from build123d import *

# Parameters (mm, degrees)
BOSS_EXTRUDE1_DEPTH   = 25.4
SKETCH2_R             = 3.5
CUT_EXTRUDE1_DEPTH    = 84.762252835
SKETCH3_R             = 13.335
CUT_EXTRUDE2_DEPTH    = 5.08
SKETCH4_R             = 22.86
CUT_EXTRUDE3_DEPTH    = 5.08
F_4_CLEARANCE_HOLE1_D = 3.2639


with BuildPart() as part:
    # Sketch1 → Boss-Extrude1 (new body)
    with BuildSketch(Plane.XY):
        with BuildLine():
            Line((-8.980256121, 56.44003455), (0, 47.459778429))
            Line((0, 47.459778429), (8.980256121, 56.44003455))
            ThreePointArc((8.980256121, 56.44003455), (21.87035816, 52.799715283), (33.559131161, 46.259131161))
            Line((33.559131161, 46.259131161), (33.559131161, 33.559131161))
            Line((33.559131161, 33.559131161), (46.259131161, 33.559131161))
            ThreePointArc((46.259131161, 33.559131161), (52.799715283, 21.87035816), (56.44003455, 8.980256121))
            Line((56.44003455, 8.980256121), (47.459778429, 0))
            Line((47.459778429, 0), (56.44003455, -8.980256121))
            ThreePointArc((56.44003455, -8.980256121), (52.799715283, -21.87035816), (46.259131161, -33.559131161))
            Line((46.259131161, -33.559131161), (33.559131161, -33.559131161))
            Line((33.559131161, -33.559131161), (33.559131161, -46.259131161))
            ThreePointArc((33.559131161, -46.259131161), (21.87035816, -52.799715283), (8.980256121, -56.44003455))
            Line((8.980256121, -56.44003455), (0, -47.459778429))
            Line((0, -47.459778429), (-8.980256121, -56.44003455))
            ThreePointArc((-8.980256121, -56.44003455), (-21.87035816, -52.799715283), (-33.559131161, -46.259131161))
            Line((-33.559131161, -46.259131161), (-33.559131161, -33.559131161))
            Line((-33.559131161, -33.559131161), (-46.259131161, -33.559131161))
            ThreePointArc((-46.259131161, -33.559131161), (-52.799715283, -21.87035816), (-56.44003455, -8.980256121))
            Line((-56.44003455, -8.980256121), (-47.459778429, 0))
            Line((-47.459778429, 0), (-56.44003455, 8.980256121))
            ThreePointArc((-56.44003455, 8.980256121), (-52.799715283, 21.87035816), (-46.259131161, 33.559131161))
            Line((-46.259131161, 33.559131161), (-33.559131161, 33.559131161))
            Line((-33.559131161, 33.559131161), (-33.559131161, 46.259131161))
            ThreePointArc((-33.559131161, 46.259131161), (-21.87035816, 52.799715283), (-8.980256121, 56.44003455))
        make_face()
    extrude(amount=BOSS_EXTRUDE1_DEPTH)

    # Sketch2 → Cut-Extrude1 (cut, through all)
    with BuildSketch(Plane.XY.offset(25.4)):
        Circle(SKETCH2_R)
    extrude(amount=-CUT_EXTRUDE1_DEPTH, mode=Mode.SUBTRACT)

    # Sketch3 → Cut-Extrude2 (cut)
    with BuildSketch(Plane.XY.offset(25.4)):
        Circle(SKETCH3_R)
    extrude(amount=-CUT_EXTRUDE2_DEPTH, mode=Mode.SUBTRACT)

    # Sketch4 → Cut-Extrude3 (cut)
    with BuildSketch(Plane(origin=(0, 0, 0), x_dir=(-1, 0, 0), z_dir=(0, 0, -1))):
        Circle(SKETCH4_R)
    extrude(amount=-CUT_EXTRUDE3_DEPTH, mode=Mode.SUBTRACT)

    # #4 Clearance Hole1 (through all)
    with Locations(Plane(origin=(0, 0, 5.08), x_dir=(-1, 0, 0), z_dir=(0, 0, -1))):
        with Locations((0, 9.525), (8.248891971, 4.7625), (8.248891971, -4.7625), (0, -9.525), (-8.248891971, 4.7625), (-8.248891971, -4.7625)):
            Hole(F_4_CLEARANCE_HOLE1_D / 2)


solid = part.part
Geometry check sheet. Reference: the model listing, model coordinates, mm. A direction names the side the tool comes from. Round coordinates to 2 decimals unless told otherwise and drop trailing zeros. Write each loop counter-clockwise with the first axis right and the second up, starting at its lowest first coordinate (ties: lowest second). Pieces come first, ordered by that corner, then holes. Notation, with made-up numbers: (87.5, -24.75) -> (146.5, -24.75) arc R13 ccw to (146.5, -19.75) -> close; hole circle Ø11 at (-4, 3). An arc over 180 degrees is marked (long way). One line per item, written item: value. Start each with the question number.
(1) Cross-section at C-C, the plane y = 37. Record the cut outline in (x, z), and give its area (3 significant figures).
(2) Draft check along X on faces 5 (the flat face through (-40, 33.559, 13)), 6 (the flat face through (-51.89, 4.43, 12.52)), 7 (the flat face through (4.55, -52.01, 12.52)). Enter one of: +X half, -X half, draft (parallel to the pull), parting line (faces both ways), or undercut.
(3) Access from +Z, -Z, +X, -X, +Y, -Y to the whole of each face (thin tool, end or side, straight path). Record for faces 1 (the flat face through (0, -5, 5.08)), 2 (the cylindrical face through (-1.74, 13.22, 22.9)), 3 (the flat face through (-33.559, -40, 13)), 4 (the flat face through (-4.55, 52.01, 12.52)).
(4) Go/stop test with flat-tipped pins: pin 1 Ø9 at (x, y) = (0, 0) entering from -Z; pin 2 Ø4 at (x, z) = (37, 11) entering from -Y; pin 3 Ø14 at (x, z) = (-40.5, 17.5) entering from +Y; pin 4 Ø5 at (x, y) = (20, 13) entering from -Z. Record where each tip stops, or that it passes through.
(5) Cross-section at B-B, the plane x = 21.5. Record the cut outline in (y, z), and give its area (3 significant figures).
(6) Cross-section at D-D, the plane z = 10. Give the number of separate pieces and of enclosed holes in the cut face, and give its area (3 significant figures).
(7) Cross-section at A-A, the plane z = 2.5. Record the cut outline in (x, y), and give its area (3 significant figures).
(8) Scan lines: line 1 (Y direction, x = 0, z = 14.5); line 2 (X direction, y = -5, z = 9.25); line 3 (Z direction, x = -15, y = 14). Record each from-to range of solid material in increasing order. Write a range as [from, to].
Answer:
1. outline: (-33.56, 0) -> (33.56, 0) -> (33.56, 25.4) -> (-33.56, 25.4) -> close
1. area: 1,700 mm²
2. face 5: draft
2. face 6: -X half
2. face 7: undercut
3. face 1: -Z
3. face 2: +Z
3. face 3: +Z, -Z, -X, -Y
3. face 4: +Z, -Z, +Y
4. pin 1: z = 5.08
4. pin 2: y = -33.56
4. pin 3: y = 46.3
4. pin 4: z = 0
5. outline: (-52.95, 0) -> (-7.77, 0) -> (-7.77, 5.08) -> (7.77, 5.08) -> (7.77, 0) -> (52.95, 0) -> (52.95, 25.4) -> (-52.95, 25.4) -> close
5. area: 2,610 mm²
6. separate pieces: 1
6. enclosed holes: 7
6. area: 9,460 mm²
7. outline: (-56.44, -8.98) arc R57.15 ccw to (-46.26, -33.56) -> (-33.56, -33.56) -> (-33.56, -46.26) arc R57.15 ccw to (-8.98, -56.44) -> (0, -47.46) -> (8.98, -56.44) arc R57.15 ccw to (33.56, -46.26) -> (33.56, -33.56) -> (46.26, -33.56) arc R57.15 ccw to (56.44, -8.98) -> (47.46, 0) -> (56.44, 8.98) arc R57.15 ccw to (46.26, 33.56) -> (33.56, 33.56) -> (33.56, 46.26) arc R57.15 ccw to (8.98, 56.44) -> (0, 47.46) -> (-8.98, 56.44) arc R57.15 ccw to (-33.56, 46.26) -> (-33.56, 33.56) -> (-46.26, 33.56) arc R57.15 ccw to (-56.44, 8.98) -> (-47.46, 0) -> close; hole circle Ø45.72 at (0, 0)
7. area: 7,910 mm²
8. line 1: [-47.46, -11.16], [-7.89, -3.5], [3.5, 7.89], [11.16, 47.46]
8. line 2: [-52.46, -9.86], [-6.63, 6.63], [9.86, 52.46]
8. line 3: [5.08, 25.4]
